The model under review builds one solid part; all positions refer to its coordinate system, in mm. A direction names the side the tool comes from. Coordinates: 2 decimals unless noted, no trailing zeros. Loops run counter-clockwise (first coordinate to the right, second up) from the corner with the lowest first, then second, coordinate; pieces in that order, holes last. Notation, with made-up numbers: M -7.75,-37.75 L 47.25,-37.75 A15 ccw 47.25,-13.75 Z; hole C 61,59.5 d5. An arc over 180 degrees is marked long. Write item = value, one per line. Start each with the question number.
Q1. For faces 1 (the face through (106.99, 4.93, 52.15)), 2 (the face through (110, 58, 10)), 3 (the face through (0, 58, 10)), 4 (the face through (96.22, 15.07, 32.505)), 5 (the face through (2.85, 16.99, 37.61)), list the 3-axis set-ups (+Z, -Z, +X, -X, +Y, -Y) from which the entire face can be reached by the end or side of a thin tool; tool diameter is ignored.
Q2. Mouldability with a two-part tool opening along Z and no side actions: class faces 6 (the face through (54, 58, 20)), 7 (the face through (54, 58, 0)), 8 (the face through (96, 10, -15)) as released by +Z, released by -Z, zero draft, split by the parting line, or undercut.
Q3. We need section B-B on z = -17.5. Give the boundary of the cut face in (x, y), and give its area (3 significant figures).
Q4. We need section D-D on y = 46.5. Give the boundary of the cut face in (x, z).
Q5. We need section C-C on y = 12. Count the separate pieces of the cut face and the enclosed holes in it, and give its area (3 significant figures).
Q6. We need section A-A on x = 14. Give the boundary of the cut face in (y, z), and give its area (3 significant figures).
Q7. Clearance check with flat-ended pins moving along their axes: pin 1 Ø16.5 at (x, z) = (70, 36) entering from +Y; pin 2 Ø6 at (x, z) = (36.5, -16) entering from -Y; pin 3 Ø11.5 at (x, z) = (14, 37.5) entering from +Y; pin 4 Ø3.5 at (x, z) = (43, 10) entering from +Y. State where each tip first meets the part, or that it passes through.
Q8. Wall thickness on probe 1 along X at (y, z) = (4.25, -17.5); probe 2 along X at (y, z) = (79, 9); probe 3 along X at (y, z) = (14, -17): over which ranges is each line inside the solid? List them lowest first.
from build123d import *

# Parameters (mm, degrees)
SKETCH2_W           = 110
SKETCH2_H           = 86
BOSS_EXTRUDE1_DEPTH = 20
SKETCH3_W           = 90
SKETCH3_H           = 20
BOSS_EXTRUDE2_DEPTH = 110
SKETCH4_R           = 1.9
CUT_EXTRUDE1_DEPTH  = 20
SKETCH5_R           = 5
CUT_EXTRUDE2_DEPTH  = 10
FILLET1_R           = 10
SKETCH6_R           = 2.1
CUT_EXTRUDE3_DEPTH  = 10


with BuildPart() as part:
    # Sketch2 → Boss-Extrude1 (new body)
    with BuildSketch(Plane.XY):
        with Locations((55, 43)):
            Rectangle(SKETCH2_W, SKETCH2_H)
    extrude(amount=BOSS_EXTRUDE1_DEPTH)

    # Sketch3 → Boss-Extrude2 (add)
    with BuildSketch(Plane(origin=(110, 0, 0), x_dir=(0, 0, -1), z_dir=(1, 0, 0))):
        with Locations((-10, 10)):
            Rectangle(SKETCH3_W, SKETCH3_H)
    extrude(amount=-BOSS_EXTRUDE2_DEPTH)

    # Sketch4 → Cut-Extrude1 (cut)
    with BuildSketch(Plane(origin=(0, 20, 0), x_dir=(1, 0, 0), z_dir=(0, 1, 0))):
        with Locations(Location((14, -37.5, 0), (0, 0, 270))):
            Circle(SKETCH4_R)
        with Locations(Location((96, -37.5, 0), (0, 0, 90))):
            Circle(SKETCH4_R)
        with Locations(Location((96, 17.5, 0), (0, 0, 270))):
            Circle(SKETCH4_R)
        with Locations(Location((14, 17.5, 0), (0, 0, 90))):
            Circle(SKETCH4_R)
    extrude(amount=-CUT_EXTRUDE1_DEPTH, mode=Mode.SUBTRACT)

    # Sketch5 → Cut-Extrude2 (cut)
    with BuildSketch(Plane(origin=(0, 20, 0), x_dir=(1, 0, 0), z_dir=(0, 1, 0))):
        with Locations(Location((96, -37.5, 0), (0, 0, 270))):
            Circle(SKETCH5_R)
        with Locations(Location((14, -37.5, 0), (0, 0, 270))):
            Circle(SKETCH5_R)
        with Locations(Location((14, 17.5, 0), (0, 0, 270))):
            Circle(SKETCH5_R)
        with Locations(Location((96, 17.5, 0), (0, 0, 270))):
            Circle(SKETCH5_R)
    extrude(amount=-CUT_EXTRUDE2_DEPTH, mode=Mode.SUBTRACT)

    # Fillet1
    # the kernel refuses this fillet: 10 mm, written as the material it adds along each edge
    with BuildSketch(Plane(origin=(0, 20, 0), x_dir=(0, 0, -1), z_dir=(1, 0, 0)), Plane(origin=(0, 20, 20), x_dir=(0, 1, 0), z_dir=(1, 0, 0))) as fillet1_piece_1:
        with BuildLine():
            CenterArc((FILLET1_R, FILLET1_R), FILLET1_R, 180, 90)
            Line((0, FILLET1_R), (0, 0))
            Line((0, 0), (FILLET1_R, 0))
        make_face()
    extrude(amount=110)
    # the kernel refuses this fillet: 10 mm, written as the material it takes off along each edge
    with BuildSketch(Plane(origin=(0, 45, -35), x_dir=(0, 0, 1), z_dir=(0, -1, 0)), Plane(origin=(110, 45, -35), x_dir=(-1, 0, 0), z_dir=(0, -1, 0)), Plane(origin=(0, -25, 55), x_dir=(0, 0, -1), z_dir=(0, 1, 0)), Plane(origin=(110, -25, 55), x_dir=(-1, 0, 0), z_dir=(0, 1, 0))) as fillet1_2_piece_1:
        with BuildLine():
            CenterArc((FILLET1_R, -FILLET1_R), FILLET1_R, 90, 90)
            Line((0, -FILLET1_R), (0, 0))
            Line((0, 0), (FILLET1_R, 0))
        make_face()
    extrude(amount=70, mode=Mode.SUBTRACT)
    with BuildSketch(Plane(origin=(135, 20, -35), x_dir=(0, -1, 0), z_dir=(-1, 0, 0))) as fillet1_2_piece_2:
        with BuildLine():
            CenterArc((FILLET1_R, FILLET1_R), FILLET1_R, 180, 90)
            Line((0, FILLET1_R), (0, 0))
            Line((0, 0), (FILLET1_R, 0))
        make_face()
    extrude(amount=160, mode=Mode.SUBTRACT)
    with BuildSketch(Plane(origin=(135, 20, 55), x_dir=(0, -1, 0), z_dir=(-1, 0, 0))) as fillet1_2_piece_3:
        with BuildLine():
            CenterArc((FILLET1_R, -FILLET1_R), FILLET1_R, 90, 90)
            Line((0, -FILLET1_R), (0, 0))
            Line((0, 0), (FILLET1_R, 0))
        make_face()
    extrude(amount=160, mode=Mode.SUBTRACT)
    # the kernel refuses this fillet: 10 mm, written as the material it takes off along each edge
    with BuildSketch(Plane(origin=(100, 10, 45), x_dir=(0, 1, 0), z_dir=(1, 0, 0))) as fillet1_3_piece_1_section:
        Polygon((0, 0), (FILLET1_R, 0), (FILLET1_R, FILLET1_R), (0, FILLET1_R), align=None)
    fillet1_3_piece_1 = extrude(amount=FILLET1_R, mode=Mode.PRIVATE)
    fillet1_3_piece_1 = fillet1_3_piece_1 - Plane(origin=(100, 10, 45), x_dir=(0, -0.7071067811865475, -0.7071067811865475), z_dir=(1, 0, 0)) * Sphere(FILLET1_R, mode=Mode.PRIVATE)
    add(fillet1_3_piece_1, mode=Mode.SUBTRACT)
    with BuildSketch(Plane(origin=(10, 10, 45), x_dir=(0, 1, 0), z_dir=(-1, 0, 0))) as fillet1_3_piece_2_section:
        Polygon((0, 0), (FILLET1_R, 0), (FILLET1_R, -FILLET1_R), (0, -FILLET1_R), align=None)
    fillet1_3_piece_2 = extrude(amount=FILLET1_R, mode=Mode.PRIVATE)
    fillet1_3_piece_2 = fillet1_3_piece_2 - Plane(origin=(10, 10, 45), x_dir=(0, -0.7071067811865475, -0.7071067811865475), z_dir=(-1, 0, 0)) * Sphere(FILLET1_R, mode=Mode.PRIVATE)
    add(fillet1_3_piece_2, mode=Mode.SUBTRACT)
    with BuildSketch(Plane(origin=(10, 10, -25), x_dir=(0, 1, 0), z_dir=(-1, 0, 0))) as fillet1_3_piece_3_section:
        Polygon((0, 0), (FILLET1_R, 0), (FILLET1_R, FILLET1_R), (0, FILLET1_R), align=None)
    fillet1_3_piece_3 = extrude(amount=FILLET1_R, mode=Mode.PRIVATE)
    fillet1_3_piece_3 = fillet1_3_piece_3 - Plane(origin=(10, 10, -25), x_dir=(0, -0.7071067811865475, 0.7071067811865475), z_dir=(-1, 0, 0)) * Sphere(FILLET1_R, mode=Mode.PRIVATE)
    add(fillet1_3_piece_3, mode=Mode.SUBTRACT)
    with BuildSketch(Plane(origin=(100, 10, -25), x_dir=(0, 1, 0), z_dir=(1, 0, 0))) as fillet1_3_piece_4_section:
        Polygon((0, 0), (FILLET1_R, 0), (FILLET1_R, -FILLET1_R), (0, -FILLET1_R), align=None)
    fillet1_3_piece_4 = extrude(amount=FILLET1_R, mode=Mode.PRIVATE)
    fillet1_3_piece_4 = fillet1_3_piece_4 - Plane(origin=(100, 10, -25), x_dir=(0, -0.7071067811865475, 0.7071067811865475), z_dir=(1, 0, 0)) * Sphere(FILLET1_R, mode=Mode.PRIVATE)
    add(fillet1_3_piece_4, mode=Mode.SUBTRACT)
    with BuildSketch(Plane(origin=(0, 111, 0), x_dir=(0, 0, 1), z_dir=(0, -1, 0)), Plane(origin=(110, 30, 0), x_dir=(0, 0, 1), z_dir=(0, 1, 0))) as fillet1_3_piece_5:
        with BuildLine():
            CenterArc((FILLET1_R, -FILLET1_R), FILLET1_R, 90, 90)
            Line((0, -FILLET1_R), (0, 0))
            Line((0, 0), (FILLET1_R, 0))
        make_face()
    extrude(amount=81, mode=Mode.SUBTRACT)
    with BuildSketch(Plane(origin=(0, 111, 20), x_dir=(0, 0, -1), z_dir=(0, -1, 0)), Plane(origin=(110, 30, 20), x_dir=(0, 0, -1), z_dir=(0, 1, 0))) as fillet1_3_piece_6:
        with BuildLine():
            CenterArc((FILLET1_R, FILLET1_R), FILLET1_R, 180, 90)
            Line((0, FILLET1_R), (0, 0))
            Line((0, 0), (FILLET1_R, 0))
        make_face()
    extrude(amount=81, mode=Mode.SUBTRACT)
    with BuildSketch(Plane(origin=(110, 20, -10), x_dir=(0, -1, 0), z_dir=(0, 0, -1)), Plane(origin=(110, 20, 45), x_dir=(0, -1, 0), z_dir=(0, 0, -1))) as fillet1_3_piece_7:
        with BuildLine():
            CenterArc((FILLET1_R, FILLET1_R), FILLET1_R, 180, 90)
            Line((0, FILLET1_R), (0, 0))
            Line((0, 0), (FILLET1_R, 0))
        make_face()
    extrude(amount=15, mode=Mode.SUBTRACT)
    with BuildSketch(Plane(origin=(0, 20, -10), x_dir=(0, -1, 0), z_dir=(0, 0, -1)), Plane(origin=(0, 20, 45), x_dir=(0, -1, 0), z_dir=(0, 0, -1))) as fillet1_3_piece_8:
        with BuildLine():
            CenterArc((FILLET1_R, -FILLET1_R), FILLET1_R, 90, 90)
            Line((0, -FILLET1_R), (0, 0))
            Line((0, 0), (FILLET1_R, 0))
        make_face()
    extrude(amount=15, mode=Mode.SUBTRACT)
    with BuildSketch(Plane(origin=(110, 30, 30), x_dir=(0, 0, -1), z_dir=(0, 1, 0))) as fillet1_3_piece_9:
        with BuildLine():
            CenterArc((10 + FILLET1_R, FILLET1_R), FILLET1_R, 180, 90)
            Line((10, FILLET1_R), (10, 0))
            Line((10, 0), (10 + FILLET1_R, 0))
        make_face()
    revolve(axis=Axis((110, 30, 30), (-1, 0, 0)), revolution_arc=90, mode=Mode.SUBTRACT)
    with BuildSketch(Plane(origin=(0, 30, 30), x_dir=(0, 0, -1), z_dir=(0, 1, 0))) as fillet1_3_piece_10:
        with BuildLine():
            CenterArc((10 + FILLET1_R, -FILLET1_R), FILLET1_R, 90, 90)
            Line((10, -FILLET1_R), (10, 0))
            Line((10, 0), (10 + FILLET1_R, 0))
        make_face()
    revolve(axis=Axis((0, 30, 30), (-1, 0, 0)), revolution_arc=90, mode=Mode.SUBTRACT)
    with BuildSketch(Plane(origin=(0, 30, -10), x_dir=(0, -1, 0), z_dir=(0, 0, -1))) as fillet1_3_piece_11:
        with BuildLine():
            CenterArc((10 + FILLET1_R, -FILLET1_R), FILLET1_R, 90, 90)
            Line((10, -FILLET1_R), (10, 0))
            Line((10, 0), (10 + FILLET1_R, 0))
        make_face()
    revolve(axis=Axis((0, 30, -10), (-1, 0, 0)), revolution_arc=90, mode=Mode.SUBTRACT)
    with BuildSketch(Plane(origin=(110, 30, -10), x_dir=(0, -1, 0), z_dir=(0, 0, -1))) as fillet1_3_piece_12:
        with BuildLine():
            CenterArc((10 + FILLET1_R, FILLET1_R), FILLET1_R, 180, 90)
            Line((10, FILLET1_R), (10, 0))
            Line((10, 0), (10 + FILLET1_R, 0))
        make_face()
    revolve(axis=Axis((110, 30, -10), (-1, 0, 0)), revolution_arc=90, mode=Mode.SUBTRACT)

    # Sketch6 → Cut-Extrude3 (cut)
    with BuildSketch(Plane(origin=(0, 86, 0), x_dir=(1, 0, 0), z_dir=(0, 1, 0))):
        with Locations(Location((18, -10, 0), (0, 0, 270))):
            Circle(SKETCH6_R)
        with Locations(Location((43, -10, 0), (0, 0, 270))):
            Circle(SKETCH6_R)
        with Locations(Location((68, -10, 0), (0, 0, 270))):
            Circle(SKETCH6_R)
        with Locations(Location((93, -10, 0), (0, 0, 270))):
            Circle(SKETCH6_R)
    extrude(amount=-CUT_EXTRUDE3_DEPTH, mode=Mode.SUBTRACT)


solid = part.part
Returned:
q1.face_1 = +Z, +X, +Y, -Y
q1.face_2 = +X, +Y
q1.face_3 = -X, +Y
q1.face_4 = +Y
q1.face_5 = +Z, -X, +Y
q2.face_6 = released by +Z
q2.face_7 = released by -Z
q2.face_8 = undercut
q3.outline = M 0,0 L 12.1,0 L 12.1,10 L 9,10 L 9,19.95 A10 ccw 0,10 Z; M 15.9,0 L 94.1,0 L 94.1,10 L 91,10 L 91,20 L 19,20 L 19,10 L 15.9,10 Z; M 97.9,0 L 110,0 L 110,10 A10 ccw 101,19.95 L 101,10 L 97.9,10 Z
q3.area = 1,880 mm^2
q4.outline = M 10,0 L 100,0 A10 ccw 100,20 L 10,20 A10 ccw Z
q5.separate_pieces = 1
q5.enclosed_holes = 4
q5.area = 9,440 mm^2
q6.outline = M 0,-35 L 10,-35 A10 ccw 20,-25 L 20,-22.5 L 10,-22.5 L 10,-19.4 L 0,-19.4 Z; M 0,-15.6 L 10,-15.6 L 10,-12.5 L 20,-12.5 L 20,-10 A10 cw 30,0 L 86,0 L 86,20 L 30,20 A10 cw 20,30 L 20,32.5 L 10,32.5 L 10,35.6 L 0,35.6 Z; M 0,39.4 L 10,39.4 L 10,42.5 L 20,42.5 L 20,45 A10 ccw 10,55 L 0,55 Z
q6.area = 2,840 mm^2
q7.pin_1 = 20.26
q7.pin_2 = 0
q7.pin_3 = 20
q7.pin_4 = 76
q8.probe_1 = 0 to 12.1, 15.9 to 94.1, 97.9 to 110
q8.probe_2 = 0.05 to 16.15, 19.85 to 41.15, 44.85 to 66.15, 69.85 to 91.15, 94.85 to 109.95
q8.probe_3 = 0.83 to 9.03, 18.97 to 91.03, 100.97 to 109.17
